The listing builds one solid part. Answer for the finished solid, in the listing's coordinates (mm). A direction names the side the tool comes from. Round coordinates to 2 decimals unless told otherwise and drop trailing zeros. Write each loop counter-clockwise with the first axis right and the second up, starting at its lowest first coordinate (ties: lowest second). Pieces come first, ordered by that corner, then holes. Notation, with made-up numbers: (15.25, -28.75) - (52.25, -28.75) arc R19 cw to (52.25, -14.75) - close; hole circle Ø8 at (-13, 23). An arc over 180 degrees is marked (long way). Return JSON: item names as keys, results as strings. Group by question number.
(1) Determine the mould class of faces 3 (the flat face through (-21, 5, -58)), 4 (the flat face through (0, 7.5, 2)), 5 (the flat face through (25, 3, 2)), 6 (the cylindrical face through (20, 3, -1)) for opening direction X: +X half, -X half, draft (parallel to the pull), parting line (faces both ways), or undercut.
(2) Find the intervals of material crossed by line 1 along Z through (x, y) = (21.25, 6.15); line 2 along Z through (x, y) = (21.25, 2.65); line 3 along X through (y, z) = (1.3, 60), in increasing order. Write a range as [from, to].
(3) Which of the six approach directions +Z, -Z, +X, -X, +Y, -Y give full straight-line access (tool end or side, diameter ignored) to faces 1 (the flat face through (-21, 5, 62)), 2 (the cylindrical face through (-22.43, 2.54, -1.08))?
(4) This flat-tipped pin is pushed along its axis until it touches: pin 1 (3.5 mm diameter, centred on x = -21.25, z = 0, fed in from +Y). Where does it stop, or does it pass through?
(5) Section A-A, the plane z = 60 is taken. Write down the section's boundary in (x, y), then the cut area to 3 significant figures.
(6) Section B-B, the plane x = 21.25 is taken. Write down the section's boundary in (y, z), then the cut area to 3 significant figures.
(7) Section C-C, the plane x = -21 is taken. Write down the section's boundary in (y, z).
Autodesk Inventor part; units mm, degrees
ref_plane "YZ Plane" through (0, 0, 0) normal (1, 0, 0) x (0, 1, 0)
ref_plane "XZ Plane" through (0, 0, 0) normal (0, 1, 0) x (-1, 0, 0)
ref_plane "XY Plane" through (0, 0, 0) normal (0, 0, 1) x (1, 0, 0)
sketch "Sketch1" plane through (0, 0, 0) normal (0, 1, 0) x (-1, 0, 0)
  line L0 (25, 63.75) -> (-25, 63.75)
  line L1 (-25, 63.75) -> (-25, -63.75)
  line L2 (-25, -63.75) -> (25, -63.75)
  line L3 (25, -63.75) -> (25, 63.75)
  point P0 (0, 0)
  dimension "d0" = 50
  dimension "d1" = 127.5
  dimension "d2" = 25
  dimension "d3" = 63.75
extrude "Extrusion1" add sketch "Sketch1" along normal blind 7.5
sketch "Sketch2" plane through (0, 7.5, 0) normal (0, 1, 0) x (1, 0, 0)
  circle A0 centre (-21.25, -60) radius 1.6
  circle A1 centre (-21.25, 60) radius 1.6
  circle A2 centre (21.25, -60) radius 1.6
  circle A3 centre (21.25, 60) radius 1.6
  circle A4 centre (-21.25, 0) radius 1.6
  circle A5 centre (21.25, 0) radius 1.6
  line L0 (25, -63.75) -> (25, 63.75)
  line L1 (25, 63.75) -> (-25, 63.75)
  line L2 (-25, -63.75) -> (25, -63.75)
  line L3 (-25, 63.75) -> (-25, -63.75)
  point P0 (0, 0)
  dimension "d6" = 3.2
  dimension "d7" = 3.2
  dimension "d8" = 3.2
  dimension "d9" = 3.2
  dimension "d10" = 3.2
  dimension "d11" = 3.2
  dimension "d12" = 3.75
  dimension "d13" = 3.75
  dimension "d14" = 3.75
  dimension "d15" = 3.75
  dimension "d16" = 3.75
  dimension "d17" = 3.75
  dimension "d18" = 3.75
  dimension "d19" = 3.75
  dimension "d20" = 3.75
  dimension "d21" = 3.75
  dimension "d22" = 63.75
  dimension "d23" = 63.75
extrude "Extrusion2" cut sketch "Sketch2" against normal through all contours A0 | A1 | A2 | A3 | A4 | A5
sketch "Sketch3" plane through (0, 7.5, 0) normal (0, 1, 0) x (1, 0, 0)
  circle A0 centre (21.25, -60) radius 1.6
  circle A1 centre (21.25, -60) radius 3.5
  circle A2 centre (21.25, 0) radius 1.6
  circle A3 centre (21.25, 0) radius 3.5
  circle A4 centre (21.25, 60) radius 3.5
  line L0 (25, 63.75) -> (-25, 63.75)
  line L1 (25, -63.75) -> (25, 63.75)
  point P0 (0, 0)
  dimension "d26" = 7
  dimension "d27" = 7
  dimension "d28" = 7
  dimension "d29" = 3.75
  dimension "d30" = 3.75
extrude "Extrusion3" cut sketch "Sketch3" against normal blind 2.5
mirror "Mirror1" about plane through (0, 0, 0) normal (1, 0, 0) of "Extrusion3"
chamfer "Chamfer1" distance 2 angle 45 3 edges at (25, 7.5, 0) (0, 7.5, -63.75) (-25, 7.5, 0)
chamfer "Chamfer2" distance 2 angle 45 2 edges at (-25, 2.75, -63.75) (25, 2.75, -63.75)
equation "\"d12\" = 0.5 * Thickness"
equation "\"d13\" = 0.5 * Thickness"
equation "\"d14\" = 0.5 * Thickness"
equation "\"d15\" = 0.5 * Thickness"
equation "\"d16\" = 0.5 * Thickness"
equation "\"d17\" = 0.5 * Thickness"
equation "\"d18\" = 0.5 * Thickness"
equation "\"d19\" = 0.5 * Thickness"
equation "\"d20\" = 0.5 * Thickness"
equation "\"d21\" = 0.5 * Thickness"
equation "\"d22\" = 0.5 * d1"
equation "\"d23\" = 0.5 * d1"
equation "\"d29\" = 0.5 * Thickness"
equation "\"d30\" = 0.5 * Thickness"
properties part number "Top Covers"
Working result:
{
 "1": {"face 3": "undercut", "face 4": "draft", "face 5": "+X half", "face 6": "undercut"},
 "2": {"line 1": "z = [-56.5, -3.5], [3.5, 56.5], [63.5, 63.75]", "line 2": "z = [-63.75, -61.6], [-58.4, -1.6], [1.6, 58.4], [61.6, 63.75]", "line 3": "x = [-25, -22.85], [-19.65, 19.65], [22.85, 25]"},
 "3": {"face 1": "+Y", "face 2": "+Y, -Y"},
 "4": {"pin 1": "stops at y = 5"},
 "5": {"outline": "(-25, 0) - (-22.85, 0) - (-22.85, 5) - (-24.75, 5) - (-24.75, 5.75) - (-25, 5.5) - close; (-19.65, 0) - (19.65, 0) - (19.65, 5) - (17.75, 5) - (17.75, 7.5) - (-17.75, 7.5) - (-17.75, 5) - (-19.65, 5) - close; (22.85, 0) - (25, 0) - (25, 5.5) - (24.75, 5.75) - (24.75, 5) - (22.85, 5) - close", "area": "307 mm^2"},
 "6": {"outline": "(0, -63.75) - (5.5, -63.75) - (5.75, -63.5) - (5, -63.5) - (5, -61.6) - (0, -61.6) - close; (0, -58.4) - (5, -58.4) - (5, -56.5) - (7.5, -56.5) - (7.5, -3.5) - (5, -3.5) - (5, -1.6) - (0, -1.6) - close; (0, 1.6) - (5, 1.6) - (5, 3.5) - (7.5, 3.5) - (7.5, 56.5) - (5, 56.5) - (5, 58.4) - (0, 58.4) - close; (0, 61.6) - (5, 61.6) - (5, 63.5) - (7.5, 63.5) - (7.5, 63.75) - (0, 63.75) - close", "area": "855 mm^2"},
 "7": {"outline": "(0, -63.75) - (5.5, -63.75) - (5.76, -63.49) - (5, -63.49) - (5, -61.58) - (0, -61.58) - close; (0, -58.42) - (5, -58.42) - (5, -56.51) - (7.5, -56.51) - (7.5, -3.49) - (5, -3.49) - (5, -1.58) - (0, -1.58) - close; (0, 1.58) - (5, 1.58) - (5, 3.49) - (7.5, 3.49) - (7.5, 56.51) - (5, 56.51) - (5, 58.42) - (0, 58.42) - close; (0, 61.58) - (5, 61.58) - (5, 63.49) - (7.5, 63.49) - (7.5, 63.75) - (0, 63.75) - close"}
}
